from build123d import *

# Parameters (mm, degrees)
BOSS_EXTRUDE1_DEPTH     = 27.56
CUT_EXTRUDE1_DEPTH      = 149.090525018
CUT_EXTRUDE1_DEPTH_BACK = 149.090525018
CUT_EXTRUDE2_DEPTH      = 149.090525174
CUT_EXTRUDE2_DEPTH_BACK = 149.090525174
SKETCH3_R               = 41.5


with BuildPart() as part:
    # Sketch1 → Boss-Extrude1 (new body)
    with BuildSketch(Plane.XY):
        with BuildLine():
            Line((22.96117968, 44), (-22.96117968, 44))
            ThreePointArc((-22.96117968, 44), (-29.323269783, 46.284832502), (-32.778097836, 52.095238095))
            ThreePointArc((-32.778097836, 52.095238095), (-89.927364847, 83.601091069), (-110.70300535, 21.738095238))
            ThreePointArc((-110.70300535, 21.738095238), (-104.55417528, 0), (-110.70300535, -21.738095238))
            ThreePointArc((-110.70300535, -21.738095238), (-89.927364847, -83.601091069), (-32.778097836, -52.095238095))
            ThreePointArc((-32.778097836, -52.095238095), (-29.323269783, -46.284832502), (-22.96117968, -44))
            Line((-22.96117968, -44), (22.96117968, -44))
            ThreePointArc((22.96117968, -44), (29.323269783, -46.284832502), (32.778097836, -52.095238095))
            ThreePointArc((32.778097836, -52.095238095), (89.927364847, -83.601091069), (110.70300535, -21.738095238))
            ThreePointArc((110.70300535, -21.738095238), (104.55417528, 0), (110.70300535, 21.738095238))
            ThreePointArc((110.70300535, 21.738095238), (89.927364847, 83.601091069), (32.778097836, 52.095238095))
            ThreePointArc((32.778097836, 52.095238095), (29.323269783, 46.284832502), (22.96117968, 44))
        make_face()
    extrude(amount=BOSS_EXTRUDE1_DEPTH)

    # Sketch2 → Cut-Extrude1 (cut, two sides: drawn at the far end of the back side and taken through both)
    with BuildSketch(Plane(origin=(0, 0, 0), x_dir=(1, 0, 0), z_dir=(0, 1, 0)).offset(-CUT_EXTRUDE1_DEPTH_BACK)):
        with BuildLine():
            Line((117, -6), (35.767564174, -6))
            ThreePointArc((35.767564174, -6), (32.945610035, -6.872461407), (31.108474327, -9.185370066))
            Line((31.108474327, -9.185370066), (26.433179694, -21.189259868))
            ThreePointArc((26.433179694, -21.189259868), (22.758908279, -25.815077185), (17.115, -27.56))
            Line((17.115, -27.56), (117, -27.56))
            Line((117, -27.56), (117, -6))
        make_face()
        with BuildLine():
            Line((-117, -27.56), (-117, -6))
            Line((-117, -6), (-35.767564174, -6))
            ThreePointArc((-35.767564174, -6), (-32.945610035, -6.872461407), (-31.108474327, -9.185370066))
            Line((-31.108474327, -9.185370066), (-26.433179694, -21.189259868))
            ThreePointArc((-26.433179694, -21.189259868), (-22.758908279, -25.815077185), (-17.115, -27.56))
            Line((-17.115, -27.56), (-117, -27.56))
        make_face()
    extrude(amount=CUT_EXTRUDE1_DEPTH + CUT_EXTRUDE1_DEPTH_BACK, mode=Mode.SUBTRACT)

    # Sketch3 → Cut-Extrude2 (cut, two sides: drawn at the far end of the back side and taken through both)
    with BuildSketch(Plane(origin=(0, 0, 0), x_dir=(-1, 0, 0), z_dir=(0, 0, -1)).offset(-CUT_EXTRUDE2_DEPTH_BACK)):
        with Locations((-74.5, 44)):
            Circle(SKETCH3_R)
        with Locations((-74.5, -44)):
            Circle(SKETCH3_R)
        with Locations((74.5, 44)):
            Circle(SKETCH3_R)
        with Locations((74.5, -44)):
            Circle(SKETCH3_R)
    extrude(amount=CUT_EXTRUDE2_DEPTH + CUT_EXTRUDE2_DEPTH_BACK, mode=Mode.SUBTRACT)

    # Cut-Sweep1: sweep along a path in Sketch4
    with BuildLine(Plane.XY.offset(27.56)) as cut_sweep1_path:
        CenterArc((0, 0), 22.5, 0, 360)
    # Sketch5 → Cut-Sweep1 (sweep, cut)
    with BuildSketch(Plane(origin=(0, 0, 0), x_dir=(0, 0, -1), z_dir=(1, 0, 0))):
        Polygon((-27.56, 22.5), (-9.185370066, 49.639215001), (-9.185370066, 86.5), (-27.56, 86.5), (-27.56, 48.201587292), align=None)
    sweep(path=cut_sweep1_path.line, mode=Mode.SUBTRACT)


solid = part.part
Could you check a few things on this model? Use its own coordinates, in mm. A direction names the side the tool comes from. Give positions to 0.01 mm unless a question says otherwise; leave off trailing zeros. Order: outer loops, then holes, each group sorted by start corner. A loop starts at its lowest first (then second) coordinate and runs counter-clockwise, first axis right, second up. Notation, with made-up numbers: (49.5, 34) -> (74.5, 34) arc R29 ccw to (74.5, 68) -> close; hole circle Ø9 at (21.25, 17.5). An arc over 180 degrees is marked (long way). Return JSON: item names as keys, results as strings.
1. I need wall thicknesses on line 1 (Y direction, x = 74.5, z = 3); line 2 (X direction, y = 35, z = 9.25); line 3 (X direction, y = -23.5, z = 8.75). Which ranges of each line are inside material? Lowest first, please. Write a range as from..to.
Answer list:
{"line 1": "y = -86.5..-85.5, -2.5..2.5, 85.5..86.5", "line 2": "x = -31.08..31.08", "line 3": "x = -31.3..31.3"}
2. Imagine slicing it at A-A on x = 74.5. List the corners of the cut face in (y, z) for me.
Answer list:
{"outline": "(-86.5, 0) -> (-85.5, 0) -> (-85.5, 6) -> (-86.5, 6) -> close; (-2.5, 0) -> (2.5, 0) -> (2.5, 6) -> (-2.5, 6) -> close; (85.5, 0) -> (86.5, 0) -> (86.5, 6) -> (85.5, 6) -> close"}
3. Imagine slicing it at B-B on y = 65. List the corners of the cut face in (x, z) for me.
Answer list:
{"outline": "(-111.45, 0) -> (-110.29, 0) -> (-110.29, 6) -> (-111.45, 6) -> close; (-38.71, 0) -> (-37.55, 0) -> (-37.55, 6) -> (-38.71, 6) -> close; (37.55, 0) -> (38.71, 0) -> (38.71, 6) -> (37.55, 6) -> close; (110.29, 0) -> (111.45, 0) -> (111.45, 6) -> (110.29, 6) -> close"}
4. Thinking about a two-plate mould opening in Y: for faces 1 (the cylindrical face through (-33.04, -42.18, 3.47)), 2 (the conical face through (-0.48, -30.22, 22.33)), 3 (the flat face through (0, 44, 6)), 4 (the cylindrical face through (36.165, 28.105, 3.466)), which applies, pulls with the +Y half, pulls with the -Y half, needs draft (parallel to the pull), parting line crosses it, or undercut?
Answer list:
{"face 1": "undercut", "face 2": "pulls with the -Y half", "face 3": "pulls with the +Y half", "face 4": "undercut"}
5. On a 3-axis mill with a long thin cutter (end or side, diameter ignored), from which of +Z, -Z, +X, -X, +Y, -Y can I reach the whole of each face in a straight line? I mean faces 5 (the cylindrical face through (29.4, 46.35, 4.53)), 6 (the cylindrical face through (-29.4, -46.35, 4.53)), 7 (the cylindrical face through (32.98, -0.86, 6.85)). Say none if no direction works.
Answer list:
{"face 5": "+Z, -Z, +Y", "face 6": "+Z, -Z, -Y", "face 7": "+Z, +X, +Y, -Y"}
6. Imagine slicing it at D-D on x = 48. List the corners of the cut face in (y, z) for me.
Answer list:
{"outline": "(-77.23, 0) -> (-75.94, 0) -> (-75.94, 6) -> (-77.23, 6) -> close; (-12.06, 0) -> (12.06, 0) -> (12.06, 6) -> (-12.06, 6) -> close; (75.94, 0) -> (77.23, 0) -> (77.23, 6) -> (75.94, 6) -> close"}
7. For pin 1 Ø2 at (y, z) = (42.5, 9) entering from -X; pin 2 Ø1.5 at (x, y) = (39, 15) entering from +Z; pin 3 Ø5 at (x, z) = (-42.5, 6) entering from -Y, each with a flat end and sliding along its axis, tell me the tip position at first contact or that it passes through.
Answer list:
{"pin 1": "stops at x = -31.77", "pin 2": "stops at z = 6", "pin 3": "stops at y = -74.59"}
8. Imagine slicing it at C-C on y = 5.5. List the corners of the cut face in (x, z) for me (3 decimals).
Answer list:
{"outline": "(-104.92, 0) -> (-89.992, 0) -> (-89.992, 6) -> (-104.92, 6) -> close; (-59.008, 0) -> (59.008, 0) -> (59.008, 6) -> (35.768, 6) arc R5 cw to (31.108, 9.185) -> (26.433, 21.189) arc R10 ccw to (17.115, 27.56) -> (-17.115, 27.56) arc R10 ccw to (-26.433, 21.189) -> (-31.108, 9.185) arc R5 cw to (-35.768, 6) -> (-59.008, 6) -> close; (89.992, 0) -> (104.92, 0) -> (104.92, 6) -> (89.992, 6) -> close"}
